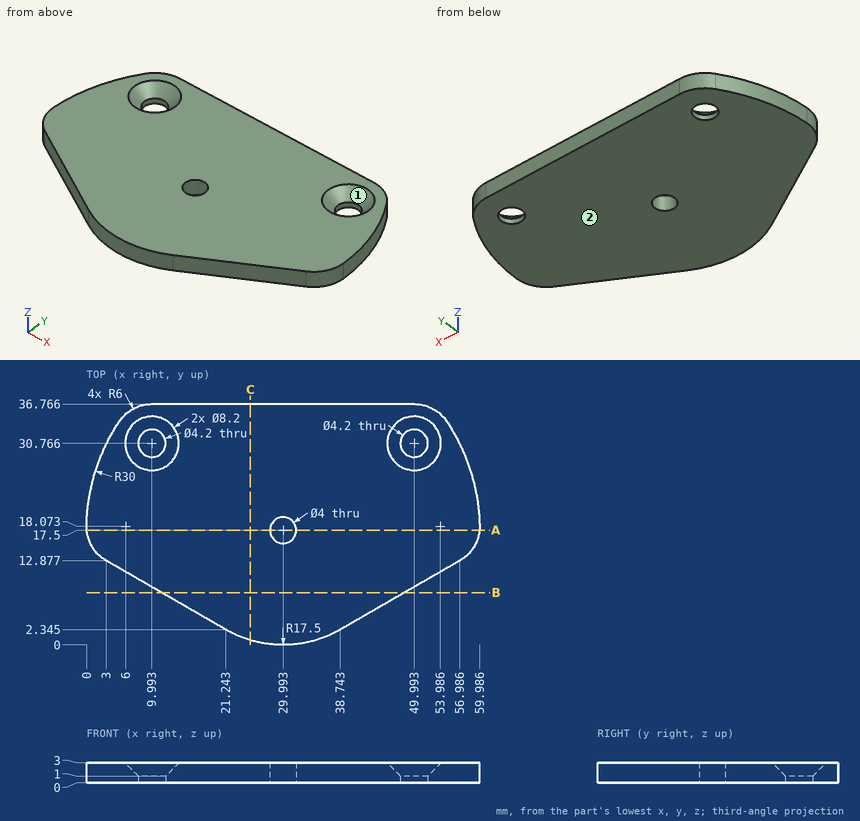
Design review of the part shown in the three views and the two pictorial views. Dimensions are in mm from the part's minimum x, y and z. Round coordinates to 2 decimals unless told otherwise and drop trailing zeros. Loops run counter-clockwise (first coordinate to the right, second up) from the corner with the lowest first, then second, coordinate; pieces in that order, holes last. Notation, with made-up numbers: (-40, 79) - (2, 79) arc R23 ccw to (2, 96) - close; hole circle Ø1 at (2, 19). An arc over 180 degrees is marked (long way). One line per item, written item: value. Start each with the question number.
Item 1: The part is to be moulded in two halves that separate along X. For the marked faces 1 and 2, say which applies: +X half, -X half, draft (parallel to the pull), parting line (faces both ways), or undercut.
Item 2: Take a section at C-C (x = 25). Give the boundary of the cut face in (y, z).
Item 3: For L1, parallel to X at y = 32, z = 1.1 (1 decimal); L2, parallel to X at y = 29.5, z = 0.8; L3, parallel to X at y = 17, z = 0.9, list the stretches that pass through material, from the lowest coordinate up.
Item 4: Clearance check with flat-ended pins moving along their axes: pin 1 Ø1 at (x, z) = (52.5, 2.5) entering from +Y; pin 2 Ø1 at (y, z) = (14.5, 0.5) entering from +X. State where each tip first meets the part, or that it passes through.
Item 5: Take a section at A-A (y = 17.5). Give the boundary of the cut face in (x, z), plus the area to 3 significant figures.
Item 6: Take a section at B-B (y = 8). Give the boundary of the cut face in (x, z).
Answer below:
1. face 1: undercut
1. face 2: draft
2. outline: (0.73, 0) - (36.77, 0) - (36.77, 3) - (0.73, 3) - close
3. L1: x = 3.7 to 8.2, 11.8 to 48.2, 51.8 to 56.3
3. L2: x = 2.5 to 8.32, 11.67 to 48.32, 51.67 to 57.49
3. L3: x = 0.1 to 28.06, 31.93 to 59.89
4. pin 1: stops at y = 36.42
4. pin 2: stops at x = 59.14
5. outline: (0.03, 0) - (27.99, 0) - (27.99, 3) - (0.03, 3) - close; (31.99, 0) - (59.96, 0) - (59.96, 3) - (31.99, 3) - close
5. area: 168 mm2
6. outline: (11.45, 0) - (48.54, 0) - (48.54, 3) - (11.45, 3) - close
